Build history of the part. All positions in model axes, mm. Face numbers are marked on the shaded views. Round coordinates to 2 decimals unless told otherwise and drop trailing zeros. Loops run counter-clockwise (first coordinate to the right, second up) from the corner with the lowest first, then second, coordinate; pieces in that order, holes last. Notation, with made-up numbers: (85, 37.5) - (135, 37.5) arc R23 ccw to (135, 55.5) - close; hole circle Ø7 at (52.5, 48.5). An arc over 180 degrees is marked (long way). Answer as CSV lines item,"result". Start each with the question number.
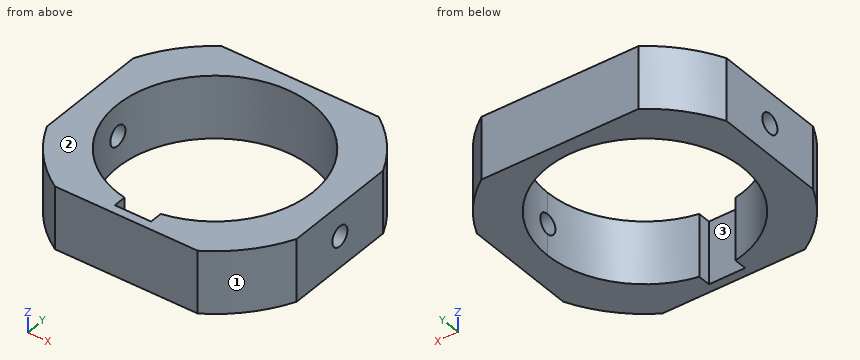
```python
from build123d import *

# Parameters (mm, degrees)
BOSS_EXTRUDE1_DEPTH     = 5
CUT_EXTRUDE1_DEPTH      = 15.933519344
CUT_EXTRUDE1_DEPTH_BACK = 15.933519344
SKETCH2_W               = 5
SKETCH2_H               = 0.5
SKETCH3_R               = 0.8
CUT_EXTRUDE2_DEPTH      = 23.657449106


with BuildPart() as part:
    # Sketch1 → Boss-Extrude1 (new body)
    with BuildSketch(Plane.XY):
        with BuildLine():
            Line((6.303155956, 9.015), (-6.303155956, 9.015))
            ThreePointArc((-6.303155956, 9.015), (-8.447474169, 7.045578767), (-10, 4.582575695))
            Line((-10, 4.582575695), (-10, -4.582575695))
            ThreePointArc((-10, -4.582575695), (-7.860673921, -7.694790803), (-4.794788838, -9.9))
            Line((-4.794788838, -9.9), (4.794788838, -9.9))
            ThreePointArc((4.794788838, -9.9), (7.860673921, -7.694790803), (10, -4.582575695))
            Line((10, -4.582575695), (10, 4.582575695))
            ThreePointArc((10, 4.582575695), (8.447474169, 7.045578767), (6.303155956, 9.015))
        make_face()
        with BuildLine():
            Line((-1.45, -8.7), (-1.45, -7.679304982))
            ThreePointArc((-1.45, -7.679304982), (-4.987107127, 6.016891847), (7.815, 0))
            ThreePointArc((7.815, 0), (6.016891847, -4.987107127), (1.45, -7.679304982))
            Line((1.45, -7.679304982), (1.45, -8.7))
            Line((1.45, -8.7), (-1.45, -8.7))
        make_face(mode=Mode.SUBTRACT)
    extrude(amount=BOSS_EXTRUDE1_DEPTH)

    # Sketch2 → Cut-Extrude1 (cut, two sides: drawn at the far end of the back side and taken through both)
    with BuildSketch(Plane(origin=(0, 0, 0), x_dir=(0, 0, -1), z_dir=(1, 0, 0)).offset(-CUT_EXTRUDE1_DEPTH_BACK)):
        with Locations((-2.5, -9.65)):
            Rectangle(SKETCH2_W, SKETCH2_H)
    extrude(amount=CUT_EXTRUDE1_DEPTH + CUT_EXTRUDE1_DEPTH_BACK, mode=Mode.SUBTRACT)

    # Sketch3 → Cut-Extrude2 (cut, through all)
    with BuildSketch(Plane(origin=(10, 0, 0), x_dir=(0, 0, -1), z_dir=(1, 0, 0))):
        with Locations(Location((-2.5, 0, 0), (0, 0, 90))):
            Circle(SKETCH3_R)
    extrude(amount=-CUT_EXTRUDE2_DEPTH, mode=Mode.SUBTRACT)


solid = part.part
```
Q1. Band-saw the part on C-C, the plane y = 3. List the corners of the cut face in (x, z).
Q2. Band-saw the part on D-D, the plane z = 3.8. List the corners of the cut face in (x, y) (3 decimals), then the cut area to 3 significant figures.
Q3. Pin check, flat tips, straight feed: pin 1 Ø4 at (x, y) = (-2.5, -7.5) entering from -Z; pin 2 Ø0.5 at (y, z) = (-8, 3) entering from +X; pin 3 Ø1 at (x, z) = (6.5, 1.5) entering from -Y; pin 4 Ø2 at (x, y) = (-6.5, -1.5) entering from -Z. Stop position of each tip, or through.
Q4. Band-saw the part on A-A, the plane z = 2.5. List the corners of the cut face in (x, y) (3 decimals), then the cut area to 3 significant figures.
Q5. Wall check: probe 1 along Z at (x, y) = (-9.25, 0); probe 2 along Y at (x, z) = (0, 3.45) (3 decimals); probe 3 along X at (y, z) = (-4.75, 2.6). Give the ranges that are in metal, low to high. Write a range as [from, to].
Q6. Band-saw the part on B-B, the plane x = 0. List the corners of the cut face in (y, z) (3 decimals), then the cut area to 3 significant figures.
Q7. Two-plate mould, pull along Y, no slides. Class the marked faces 1, 2 and 3: released by +Y, released by -Y, zero draft, split by the parting line, or undercut.
Reported:
1,outline,"(-10, 0) - (-7.22, 0) - (-7.22, 5) - (-10, 5) - close; (7.22, 0) - (10, 0) - (10, 5) - (7.22, 5) - close"
2,outline,"(-10, -4.583) arc R11 ccw to (-5.713, -9.4) - (5.713, -9.4) arc R11 ccw to (10, -4.583) - (10, 4.583) arc R11 ccw to (6.303, 9.015) - (-6.303, 9.015) arc R11 ccw to (-10, 4.583) - close; hole (-1.45, -8.7) - (1.45, -8.7) - (1.45, -7.679) arc R7.815 ccw (long way) to (-1.45, -7.679) - close"
2,area,"144 mm2"
3,pin 1,"stops at z = 0"
3,pin 2,"stops at x = 7.81"
3,pin 3,"stops at y = -9.22"
3,pin 4,"passes through"
4,outline,"(-10, -4.583) arc R11 ccw to (-5.713, -9.4) - (5.713, -9.4) arc R11 ccw to (10, -4.583) - (10, -0.8) - (7.774, -0.8) arc R7.815 cw to (1.45, -7.679) - (1.45, -8.7) - (-1.45, -8.7) - (-1.45, -7.679) arc R7.815 cw to (-7.774, -0.8) - (-10, -0.8) - close; (-10, 0.8) - (-7.774, 0.8) arc R7.815 cw to (7.774, 0.8) - (10, 0.8) - (10, 4.583) arc R11 ccw to (6.303, 9.015) - (-6.303, 9.015) arc R11 ccw to (-10, 4.583) - close"
4,area,"137 mm2"
5,probe 1,"z = [0, 1.7], [3.3, 5]"
5,probe 2,"y = [-9.4, -8.7], [7.815, 9.015]"
5,probe 3,"x = [-9.92, -6.21], [6.21, 9.92]"
6,outline,"(-9.4, 0) - (-8.7, 0) - (-8.7, 5) - (-9.4, 5) - close; (7.815, 0) - (9.015, 0) - (9.015, 5) - (7.815, 5) - close"
6,area,"9.50 mm2"
7,face 1,"released by -Y"
7,face 2,"zero draft"
7,face 3,"undercut"
